Job drawing, mm, ordinate dimensions from the low corner. One solid piece. A direction names the side the tool comes from. Round coordinates to 2 decimals unless told otherwise and drop trailing zeros. Loops run counter-clockwise (first coordinate to the right, second up) from the corner with the lowest first, then second, coordinate; pieces in that order, holes last.
1) Band-saw the part on B-B, the plane y = 7.25. Write the cut outline in (x, z).
2) Mould opens along X. For the marked faces 1, 2 and 3 say: +X half, -X half, draft (parallel to the pull), parting line (faces both ways), or undercut.
3) Drop flat-ended pins along their axis: P1, Ø1.6, axis at x = 4.5, z = 15, coming from the +Y side; P2, Ø5, axis at x = 4.5, z = 8.5, coming from the +Y side; P3, Ø7, axis at x = 32, z = 6.5, coming from the +Y side. Give the stop position or say it passes through.
4) 3-axis set-ups, long thin cutter, end or side, ignore diameter. For the marked faces 4, 5, 6, 7 and 8: which of +Z, -Z, +X, -X, +Y, -Y reach the whole face in a straight line?
5) Band-saw the part on C-C, the plane z = 18.75. Write the cut outline in (x, y), then the cut area to 3 significant figures.
6) Probe line 1 (Z direction, x = 31.5, y = 1.5); line 2 (Z direction, x = 5, y = 1); line 3 (Y direction, x = 30, z = 6). List the from-to ranges inside material, lowest first.
7) Band-saw the part on A-A, the plane z = 5. Write the cut outline in (x, y), then the cut area to 3 significant figures.
8) Band-saw the part on D-D, the plane x = 18. Write the cut outline in (y, z), then the cut area to 3 significant figures.
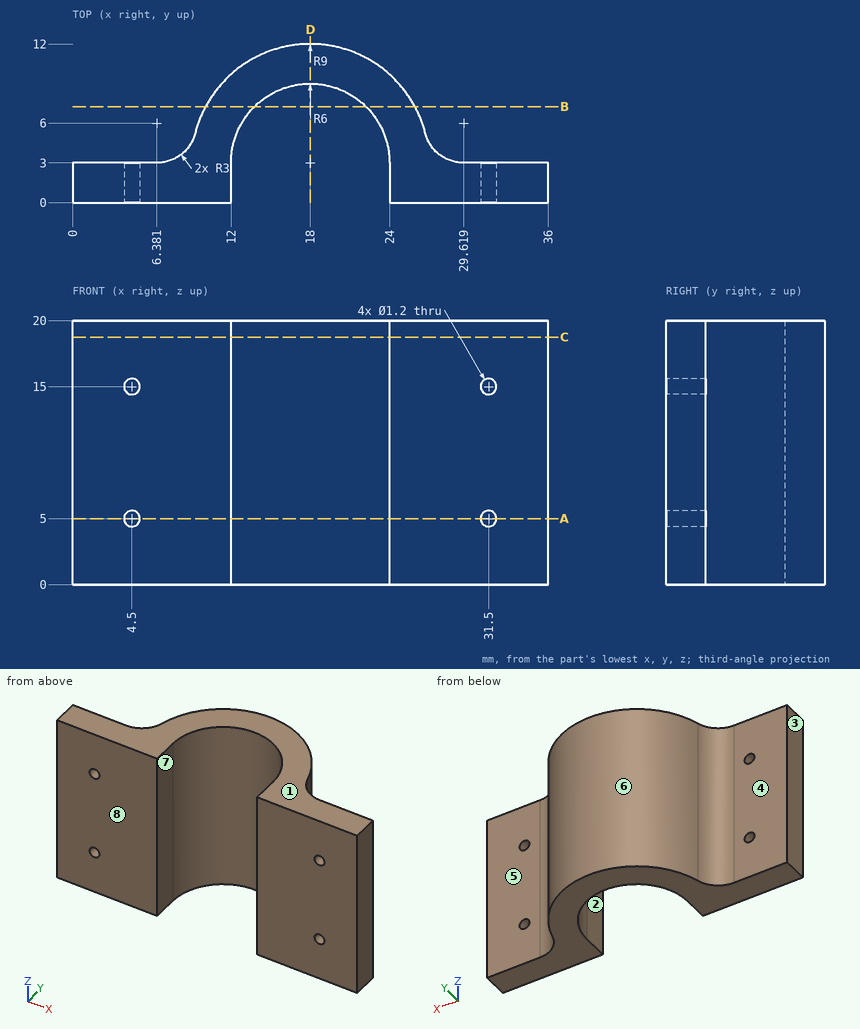
Reported:
1. outline: (10.07, 0) - (13.76, 0) - (13.76, 20) - (10.07, 20) - close; (22.24, 0) - (25.93, 0) - (25.93, 20) - (22.24, 20) - close
2. face 1: draft
2. face 2: undercut
2. face 3: -X half
3. P1: stops at y = 3
3. P2: stops at y = 3.06
3. P3: stops at y = 3.22
4. face 4: +Z, -Z, -X, +Y
4. face 5: +Z, -Z, +X, +Y
4. face 6: +Z, -Z, +Y
4. face 7: +Z, -Z, -Y
4. face 8: +Z, -Z, +X, -X, -Y
5. outline: (0, 0) - (12, 0) - (12, 3) arc R6 cw to (24, 3) - (24, 0) - (36, 0) - (36, 3) - (29.62, 3) arc R3 cw to (26.71, 5.25) arc R9 ccw to (9.29, 5.25) arc R3 cw to (6.38, 3) - (0, 3) - close
5. area: 145 mm2
6. line 1: z = 0 to 4.4, 5.6 to 14.4, 15.6 to 20
6. line 2: z = 0 to 4.67, 5.33 to 14.67, 15.33 to 20
6. line 3: y = 0 to 3
7. outline: (0, 0) - (3.9, 0) - (3.9, 3) - (0, 3) - close; (5.1, 0) - (12, 0) - (12, 3) arc R6 cw to (24, 3) - (24, 0) - (30.9, 0) - (30.9, 3) - (29.62, 3) arc R3 cw to (26.71, 5.25) arc R9 ccw to (9.29, 5.25) arc R3 cw to (6.38, 3) - (5.1, 3) - close; (32.1, 0) - (36, 0) - (36, 3) - (32.1, 3) - close
7. area: 138 mm2
8. outline: (9, 0) - (12, 0) - (12, 20) - (9, 20) - close
8. area: 60.0 mm2
